The listing builds one solid part. Answer for the finished solid, in the listing's coordinates (mm). Face numbers are marked on the shaded views. Coordinates: 2 decimals unless noted, no trailing zeros. Order: outer loops, then holes, each group sorted by start corner. A loop starts at its lowest first (then second) coordinate and runs counter-clockwise, first axis right, second up. Notation, with made-up numbers: (-10, -35.5) -> (13, -35.5) arc R18 ccw to (13, -29.5) -> close; hole circle Ø10 at (11.5, -9.75). An arc over 180 degrees is marked (long way). Answer in a Markdown table with one row per item. Add a question column.
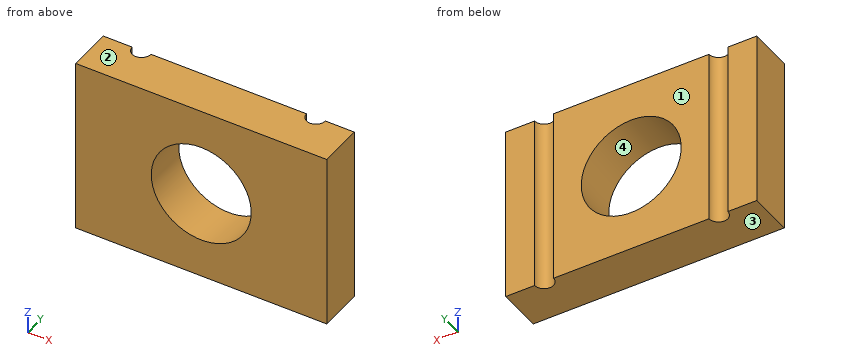
```python
from build123d import *

# Parameters (mm, degrees)
SKETCH1_W           = 35.8902
SKETCH1_H           = 25.4
SKETCH1_R           = 7.14375
BOSS_EXTRUDE1_DEPTH = 6.35
SKETCH2_R           = 1.3462
CUT_EXTRUDE1_DEPTH  = 32.741284064


with BuildPart() as part:
    # Sketch1 → Boss-Extrude1 (new body)
    with BuildSketch(Plane(origin=(0, 0, 0), x_dir=(1, 0, 0), z_dir=(0, 1, 0))):
        Rectangle(SKETCH1_W, SKETCH1_H)
        with Locations(Location((0, 0, 0), (0, 0, 270))):
            Circle(SKETCH1_R, mode=Mode.SUBTRACT)
    extrude(amount=BOSS_EXTRUDE1_DEPTH)

    # Sketch2 → Cut-Extrude1 (cut, through all)
    with BuildSketch(Plane.XY.offset(12.7)):
        with Locations((-12.4587, 6.35)):
            Circle(SKETCH2_R)
        with Locations((12.4587, 6.35)):
            Circle(SKETCH2_R)
    extrude(amount=-CUT_EXTRUDE1_DEPTH, mode=Mode.SUBTRACT)


solid = part.part
```
Q1. A cutting plane is placed at A-A (x = 0). Determine the outline of the cut face in (y, z).
Q2. Straight lines are drawn through the part: line 1 (X direction, y = 4.25, z = 0); line 2 (X direction, y = 5.75, z = 6); line 3 (X direction, y = 0.5, z = -3.5). For each, find the intervals that lie inside material, in ascending order.
Q3. A cutting plane is placed at B-B (z = 1.75). Determine the outline of the cut face in (x, y).
Q4. A cutting plane is placed at D-D (z = -1.25). Determine the outline of the cut face in (x, y).
Q5. Given pin 1 (1 mm diameter, centred on x = 4, z = 2.5, fed in from -Y), flat-ended and moving along its own axis, determine where the tip first touches the part or whether it passes through.
Q6. Determine the mould class of the marked faces 1, 2, 3 and 4 for opening direction Z: +Z half, -Z half, draft (parallel to the pull), parting line (faces both ways), or undercut.
Q7. A cutting plane is placed at C-C (y = 3.75). Determine the outline of the cut face in (x, z).
Returned:
| question | item | result |
|---|---|---|
| 1 | outline | (0, -12.7) -> (6.35, -12.7) -> (6.35, -7.14) -> (0, -7.14) -> close; (0, 7.14) -> (6.35, 7.14) -> (6.35, 12.7) -> (0, 12.7) -> close |
| 2 | line 1 | x = -17.95 to -7.14, 7.14 to 17.95 |
| 2 | line 2 | x = -17.95 to -13.66, -11.25 to -3.88, 3.88 to 11.25, 13.66 to 17.95 |
| 2 | line 3 | x = -17.95 to -6.23, 6.23 to 17.95 |
| 3 | outline | (-17.95, 0) -> (-6.93, 0) -> (-6.93, 6.35) -> (-11.11, 6.35) arc R1.35 cw to (-13.8, 6.35) -> (-17.95, 6.35) -> close; (6.93, 0) -> (17.95, 0) -> (17.95, 6.35) -> (13.8, 6.35) arc R1.35 cw to (11.11, 6.35) -> (6.93, 6.35) -> close |
| 4 | outline | (-17.95, 0) -> (-7.03, 0) -> (-7.03, 6.35) -> (-11.11, 6.35) arc R1.35 cw to (-13.8, 6.35) -> (-17.95, 6.35) -> close; (7.03, 0) -> (17.95, 0) -> (17.95, 6.35) -> (13.8, 6.35) arc R1.35 cw to (11.11, 6.35) -> (7.03, 6.35) -> close |
| 5 | pin 1 | passes through |
| 6 | face 1 | draft |
| 6 | face 2 | +Z half |
| 6 | face 3 | -Z half |
| 6 | face 4 | undercut |
| 7 | outline | (-17.95, -12.7) -> (17.95, -12.7) -> (17.95, 12.7) -> (-17.95, 12.7) -> close; hole circle Ø14.29 at (0, 0) |
